```python
from build123d import *

# Parameters (mm, degrees)
F1_DEPTH       = 18.5
F2_DEPTH       = 6.5
F3_DEPTH       = 1.5
F4_DEPTH       = 13.5
F6_D           = 4.5
F6_DEPTH       = 7
F6_CSINK_D     = 9
F6_CSINK_ANGLE = 90


with BuildPart() as f1:
    # F0 (on Front) → F1 (new body, symmetric)
    with BuildSketch(Plane.XZ):
        with BuildLine():
            Line((-8.603998, 19.092317), (2.646002, 19.092317))
            ThreePointArc((2.646002, 19.092317), (6.266849, 20.096509), (8.853265, 22.822198))
            ThreePointArc((8.853265, 22.822198), (9.676002, 26.122317), (8.853265, 29.422437))
            ThreePointArc((8.853265, 29.422437), (6.266849, 32.148126), (2.646002, 33.152317))
            Line((2.646002, 33.152317), (-19.053998, 33.152317))
            ThreePointArc((-19.053998, 33.152317), (-19.619683, 32.918003), (-19.853998, 32.352317))
            Line((-19.853998, 32.352317), (-19.853998, 29.922317))
            ThreePointArc((-19.853998, 29.922317), (-19.619683, 29.356632), (-19.053998, 29.122317))
            Line((-19.053998, 29.122317), (2.646002, 29.122317))
            ThreePointArc((2.646002, 29.122317), (5.646002, 26.122317), (2.646002, 23.122317))
            Line((2.646002, 23.122317), (-19.053998, 23.122317))
            ThreePointArc((-19.053998, 23.122317), (-19.619683, 22.888003), (-19.853998, 22.322317))
            Line((-19.853998, 22.322317), (-19.853998, 19.892317))
            ThreePointArc((-19.853998, 19.892317), (-19.619683, 19.326632), (-19.053998, 19.092317))
            Line((-19.053998, 19.092317), (-12.603998, 19.092317))
            Line((-12.603998, 19.092317), (-8.603998, 19.092317))
        make_face()
    extrude(amount=F1_DEPTH, both=True)

    # F0 (on Front) → F2 (join, symmetric)
    with BuildSketch(Plane.XZ):
        with BuildLine():
            ThreePointArc((8.853265, 29.422437), (9.676002, 26.122317), (8.853265, 22.822198))
            Line((8.853265, 22.822198), (12.856312, 23.211387))
            ThreePointArc((12.856312, 23.211387), (11.92159, 26.122317), (12.856312, 29.033247))
            Line((12.856312, 29.033247), (8.853265, 29.422437))
        make_face()
        with BuildLine():
            ThreePointArc((12.856312, 29.033247), (11.92159, 26.122317), (12.856312, 23.211387))
            ThreePointArc((12.856312, 23.211387), (17.102599, 21.125595), (21.186836, 23.513164))
            Line((21.186836, 23.513164), (19.677439, 23.964703))
            ThreePointArc((19.677439, 23.964703), (13.424495, 25.979745), (19.492658, 28.497104))
            Line((19.492658, 28.497104), (20.773135, 29.310671))
            ThreePointArc((20.773135, 29.310671), (19.539969, 30.381905), (18.027346, 30.998515))
            ThreePointArc((18.027346, 30.998515), (16.92159, 31.122317), (15.815834, 30.998515))
            ThreePointArc((15.815834, 30.998515), (14.155642, 30.287594), (12.856312, 29.033247))
        make_face()
    extrude(amount=F2_DEPTH, both=True)

    # F0 (on Front) → F3 (join, symmetric)
    with BuildSketch(Plane.XZ):
        with BuildLine():
            Line((15.815834, 36.198515), (15.815834, 30.998515))
            ThreePointArc((15.815834, 30.998515), (16.92159, 31.122317), (18.027346, 30.998515))
            Line((18.027346, 30.998515), (18.027346, 36.198515))
            ThreePointArc((18.027346, 36.198515), (17.793031, 36.7642), (17.227346, 36.998515))
            Line((17.227346, 36.998515), (16.615834, 36.998515))
            ThreePointArc((16.615834, 36.998515), (16.050149, 36.7642), (15.815834, 36.198515))
        make_face()
    extrude(amount=F3_DEPTH, both=True)

    # F0 (on Front) → F4 (join, symmetric)
    with BuildSketch(Plane.XZ):
        with BuildLine():
            Line((-13.68744, 1.668259), (-8.603998, 19.092317))
            Line((-8.603998, 19.092317), (-12.603998, 19.092317))
            Line((-12.603998, 19.092317), (-17.556703, 2.116375))
            ThreePointArc((-17.556703, 2.116375), (-17.428738, 1.412341), (-16.78872, 1.092317))
            Line((-16.78872, 1.092317), (-14.455423, 1.092317))
            ThreePointArc((-14.455423, 1.092317), (-13.975447, 1.252299), (-13.68744, 1.668259))
        make_face()
    extrude(amount=F4_DEPTH, both=True)

    # F6
    with Locations(Plane.XY.offset(33.152317)):
        with Locations((-9.603998, 10), (-9.603998, -10)):
            CounterSinkHole(F6_D / 2, F6_CSINK_D / 2, depth=F6_DEPTH, counter_sink_angle=F6_CSINK_ANGLE)


solid = f1.part
```
Model file for the job. Use its own axes, mm. A direction names the side the tool comes from. Round coordinates to 2 decimals unless told otherwise and drop trailing zeros. Write each loop counter-clockwise with the first axis right and the second up, starting at its lowest first coordinate (ties: lowest second). Pieces come first, ordered by that corner, then holes. Notation, with made-up numbers: (30.25, 37) - (39.25, 37) arc R13 cw to (39.25, 62) - close; hole circle Ø1 at (55, 59.25). An arc over 180 degrees is marked (long way). One line per item, written item: value.
(1) Drop flat-ended pins along their axis: P1, Ø2.5, axis at x = -13, z = 13, coming from the +Y side; P2, Ø2.5, axis at y = -0.5, z = 34.5, coming from the -X side; P3, Ø6.5, axis at x = 16.92, z = 26.12, coming from the +Y side; P4, Ø0.7, axis at x = 16.5, z = 33.5, coming from the -Y side. Give the stop position or say it passes through.
Values follow:
P1: stops at y = 13.5
P2: stops at x = 15.82
P3: passes through
P4: stops at y = -1.5
(2) Cut at D-D, the plane x = 11.5. Give the cut face in (y, z).
Values follow:
outline: (-6.5, 23.08) - (6.5, 23.08) - (6.5, 29.17) - (-6.5, 29.17) - close
(3) Cut at A-A, the plane y = -10. Give the cut face in (x, z).
Values follow:
outline: (-19.85, 19.89) arc R0.8 ccw to (-19.05, 19.09) - (-12.6, 19.09) - (-17.56, 2.12) arc R0.8 ccw to (-16.79, 1.09) - (-14.46, 1.09) arc R0.8 ccw to (-13.69, 1.67) - (-8.6, 19.09) - (2.65, 19.09) arc R7.03 ccw to (8.85, 22.82) arc R7.03 ccw to (8.85, 29.42) arc R7.03 ccw to (2.65, 33.15) - (-5.1, 33.15) - (-7.35, 30.9) - (-7.35, 29.12) - (2.65, 29.12) arc R3 cw to (2.65, 23.12) - (-19.05, 23.12) arc R0.8 ccw to (-19.85, 22.32) - close; (-19.85, 29.92) arc R0.8 ccw to (-19.05, 29.12) - (-11.85, 29.12) - (-11.85, 30.9) - (-14.1, 33.15) - (-19.05, 33.15) arc R0.8 ccw to (-19.85, 32.35) - close
(4) Cut at B-B, the plane x = 1. Give the cut face in (y, z), plus the area to 3 significant figures.
Values follow:
outline: (-18.5, 19.09) - (18.5, 19.09) - (18.5, 23.12) - (-18.5, 23.12) - close; (-18.5, 29.12) - (18.5, 29.12) - (18.5, 33.15) - (-18.5, 33.15) - close
area: 298 mm²
(5) Two-plate mould, pull along X, no slides. Class faces 1 (the conical face through (-9.09, -12.3, 31.01)), 2 (the cylindrical face through (-17.435, -0.189, 1.421)), 3 (the cylindrical face through (-10.81, -8.1, 30)), 4 (the flat face through (-16, 0, 1.092)): pulls with the +X half, pulls with the -X half, needs draft (parallel to the pull), parting line crosses it, or undercut.
Values follow:
face 1: undercut
face 2: pulls with the -X half
face 3: undercut
face 4: needs draft
(6) Wall check: probe 1 along Z at (x, y) = (-4.5, -7.5); probe 2 along Z at (x, y) = (15, -2); probe 3 along X at (y, z) = (-10, 30). Give the ranges that are in metal, low to high.
Values follow:
probe 1: z = 19.09 to 23.12, 29.12 to 33.15
probe 2: z = 21.51 to 23.2, 29.05 to 30.74
probe 3: x = -19.85 to -11.85, -7.35 to 8.51
(7) 3-axis set-ups, long thin cutter, end or side, ignore diameter. For faces 5 (the cylindrical face through (-10.81, 11.9, 30)), 6 (the flat face through (-8, 0, 23.122)), 7 (the flat face through (20.124, -0.091, 28.898)): which of +Z, -Z, +X, -X, +Y, -Y reach the whole face in a straight line?
Values follow:
face 5: +Z
face 6: -X, +Y, -Y
face 7: +X, +Y, -Y
(8) Cut at C-C, the plane z = 25. Give the cut face in (x, y), plus the area to 3 significant figures.
Values follow:
outline: (5.43, -18.5) - (9.59, -18.5) - (9.59, -6.5) - (13.61, -6.5) - (13.61, 6.5) - (9.59, 6.5) - (9.59, 18.5) - (5.43, 18.5) - close
area: 206 mm²
